The model under review builds one solid part; all positions refer to its coordinate system, in mm. A direction names the side the tool comes from. Coordinates: 2 decimals unless noted, no trailing zeros. Loops run counter-clockwise (first coordinate to the right, second up) from the corner with the lowest first, then second, coordinate; pieces in that order, holes last. Notation, with made-up numbers: M 33.25,29 L 73.25,29 A32 ccw 73.25,58 Z; hole C -21,67.25 d10. An arc over 180 degrees is marked long. Return JSON: item names as keys, results as strings.
Autodesk Inventor part; units mm, degrees
ref_plane "Work Plane1" through (0, 0, -3) normal (0, 0, 1) x (1, 0, 0)
ref_plane "Work Plane2" through (0, 0, 4) normal (0, 0, 1) x (1, 0, 0)
ref_plane "Work Plane3" through (0, 0, -3) normal (0, 0, 1) x (1, 0, 0)
ref_plane "Work Plane1" through (0, 0, -3) normal (0, 0, 1) x (1, 0, 0)
sketch "Sketch1" plane through (0, 0, -3) normal (0, 0, 1) x (1, 0, 0)
  circle A0 centre (0, 0) radius 2.75
extrude "M3_Head_Envelope" add sketch "Sketch1" along normal blind 3
sketch "Sketch2" plane through (0, 0, 0) normal (0, 0, 1) x (1, 0, 0)
  circle A0 centre (0, 0) radius 1.5
extrude "M3_Clearance_Grip" add sketch "Sketch2" along normal blind 4
ref_plane "Work Plane2" through (0, 0, 4) normal (0, 0, 1) x (1, 0, 0)
sketch "Sketch3" plane through (0, 0, 4) normal (0, 0, 1) x (1, 0, 0)
  circle A0 centre (0, 0) radius 1.5
extrude "Thread_Core_No_Helix" add sketch "Sketch3" along normal blind 4
ref_plane "Work Plane3" through (0, 0, -3) normal (0, 0, 1) x (1, 0, 0)
sketch "Sketch4" plane through (0, 0, -3) normal (0, 0, 1) x (1, 0, 0)
  circle A0 centre (0, 0) radius 1.25
extrude "Extrusion4" cut sketch "Sketch4" along normal blind 1.5
properties part number "Rod_M3x8_Simplified"
1. The part is to be moulded in two halves that separate along X. For faces 3 (the face through (1.2, -1.2, 0)), 4 (the face through (-0.27, 1.22, -2.26)), 5 (the face through (-1.5, -0.07, 3.94)), say which applies: released by +X, released by -X, zero draft, split by the parting line, or undercut.
Check values:
{"face 3": "zero draft", "face 4": "undercut", "face 5": "split by the parting line"}
2. To check wall thickness, follow line 1 (Y direction, x = 0, z = -2.25); line 2 (X direction, y = -0.1, z = 7.5); line 3 (Z direction, x = 0.8, y = 0.1). State the ranges of each line that lie inside material, in increasing order.
Check values:
{"line 1": "-2.75 to -1.25, 1.25 to 2.75", "line 2": "-1.5 to 1.5", "line 3": "-1.5 to 8"}
3. Add section C-C on z = -1.25. Give the boundary of the cut face in (x, y).
Check values:
{"outline": "C 0,0 d5.5"}
4. Add section D-D on z = 2.75. Give the boundary of the cut face in (x, y).
Check values:
{"outline": "C 0,0 d3"}
5. Machinability: for faces 1 (the face through (-0.596, 2.685, -1.521)), 2 (the face through (0, 0, -1.5)), which of the approach directions +Z, -Z, +X, -X, +Y, -Y give a long, thin tool a straight path to every point of the face, cutting with its end or side? Answer none if there is none.
Check values:
{"face 1": "+Z, -Z", "face 2": "-Z"}
6. Add section A-A on y = 0. Give the boundary of the cut face in (x, z).
Check values:
{"outline": "M -2.75,-3 L -1.25,-3 L -1.25,-1.5 L 1.25,-1.5 L 1.25,-3 L 2.75,-3 L 2.75,0 L 1.5,0 L 1.5,8 L -1.5,8 L -1.5,0 L -2.75,0 Z"}
7. Insertion check: pin 1 Ø2 at (x, y) = (0.5, -0.5) entering from -Z; pin 2 Ø2 at (y, z) = (2, 3) entering from -X; pin 3 Ø1 at (x, z) = (-1.5, 3.5) entering from +Y. Each pin has a flat end and moves straight along its axis. Give the tip position at first contact, or say it passes through.
Check values:
{"pin 1": "z = -3", "pin 2": "x = -1.12", "pin 3": "y = 1.12"}
